```python
from build123d import *

# Parameters (mm, degrees)
SKETCH1_R               = 40
SKETCH1_R_2             = 14
BOSS_EXTRUDE1_DEPTH     = 10
SKETCH2_W               = 16
SKETCH2_H               = 60.808164115
BOSS_EXTRUDE2_DEPTH     = 10
FILLET1_R               = 4
SKETCH3_W               = 14.5
SKETCH3_H               = 2
SKETCH4_W               = 1.3
SKETCH4_H               = 0.7
CUT_EXTRUDE1_DEPTH      = 109.166538264
CUT_EXTRUDE1_DEPTH_BACK = 109.166538264
SKETCH5_W               = 2
SKETCH5_H               = 50


with BuildPart() as part:
    # Sketch1 → Boss-Extrude1 (new, symmetric)
    with BuildSketch(Plane.XY):
        Circle(SKETCH1_R)
        Circle(SKETCH1_R_2, mode=Mode.SUBTRACT)
    extrude(amount=BOSS_EXTRUDE1_DEPTH, both=True)

    # Sketch2 → Boss-Extrude2 (add, symmetric)
    with BuildSketch(Plane.XY):
        with Locations((0, 69.595917942)):
            Rectangle(SKETCH2_W, SKETCH2_H)
    extrude(amount=BOSS_EXTRUDE2_DEPTH, both=True)

    # Fillet1
    fillet1_edges = [part.edges().sort_by_distance(p)[0] for p in [
        (-8, 39.191835885, 0),
        (8, 39.191835885, 0),
    ]]
    fillet(fillet1_edges, radius=FILLET1_R)

    # Sketch3 → Cut-Revolve1 (revolve, cut)
    with BuildSketch(Plane(origin=(0, 0, 0), x_dir=(0, 0, -1), z_dir=(1, 0, 0)), mode=Mode.PRIVATE) as cut_revolve1_sk:
        with Locations((-2.75, 15)):
            Rectangle(SKETCH3_W, SKETCH3_H)
    revolve(cut_revolve1_sk.sketch.rotate(Axis((0, 0, 0), (0, 0, -1)), 90), axis=Axis((0, 0, 0), (0, 0, -1)), mode=Mode.SUBTRACT)

    # Sketch4 → Cut-Revolve2 (revolve, cut)
    with BuildSketch(Plane(origin=(0, 0, 0), x_dir=(0, 0, -1), z_dir=(1, 0, 0)), mode=Mode.PRIVATE) as cut_revolve2_sk:
        with Locations((-5.05, 16.35)):
            Rectangle(SKETCH4_W, SKETCH4_H)
    revolve(cut_revolve2_sk.sketch.rotate(Axis((0, 0, 0), (0, 0, -1)), 90), axis=Axis((0, 0, 0), (0, 0, -1)), mode=Mode.SUBTRACT)

    # Sketch5 → Cut-Extrude1 (cut, two sides: drawn at the far end of the back side and taken through both)
    with BuildSketch(Plane(origin=(0, 0, 0), x_dir=(0, 0, -1), z_dir=(1, 0, 0)).offset(-CUT_EXTRUDE1_DEPTH_BACK)):
        with Locations((9, 75)):
            Rectangle(SKETCH5_W, SKETCH5_H)
        with Locations((-9, 75)):
            Rectangle(SKETCH5_W, SKETCH5_H)
    extrude(amount=CUT_EXTRUDE1_DEPTH + CUT_EXTRUDE1_DEPTH_BACK, mode=Mode.SUBTRACT)


solid = part.part
```
Check sheet for the modelled part. Datum: model origin and axes. Units: mm. A direction names the side the tool comes from. Round coordinates to 2 decimals unless told otherwise and drop trailing zeros. Order: outer loops, then holes, each group sorted by start corner. A loop starts at its lowest first (then second) coordinate and runs counter-clockwise, first axis right, second up. Notation, with made-up numbers: (68.5, -3) -> (83.5, -3) arc R21 cw to (83.5, 8) -> close; hole circle Ø8 at (52.25, 31.25). An arc over 180 degrees is marked (long way). One line per item, written item: value. Start each with the question number.
Q1. Set-up check for faces 1 (the face through (-8, 71, 0)), 2 (the face through (0.07, 14.15, -4.5)), 3 (the face through (8, 71, 0)): record each of +Z, -Z, +X, -X, +Y, -Y from which the full face is reachable in a straight line by a thin tool's end or side.
Q2. Cross-section at C-C (y = 0). Record the boundary of the cut face in (x, z).
Q3. Cross-section at A-A (z = 1.5). Record the boundary of the cut face in (x, y), and give its area (3 significant figures).
Q4. Cross-section at B-B (x = 0). Record the boundary of the cut face in (y, z), and give its area (3 significant figures).
Q5. Cross-section at D-D (y = 58). Record the boundary of the cut face in (x, z), and give its area (3 significant figures).
Q6. Mould release check, pull along Z, two halves, no side actions. Record for faces 4 (the face through (8, 16, 10)), 5 (the face through (0, 75, -8)), 6 (the face through (-2.17, -16.56, 5.04)), 7 (the face through (-3.47, 15.62, 7.82)): pulls with the +Z half, pulls with the -Z half, needs draft (parallel to the pull), parting line crosses it, or undercut.
Q7. Thickness scan on line 1 (X direction, y = 0, z = -8.6); line 2 (Y direction, x = 0, z = 4.9); line 3 (X direction, y = 1, z = -0.25). Record the ranges inside material, lowest first.
Q8. Gauge pin test, flat ends, axial feed: pin 1 Ø6 at (y, z) = (70.5, -5) entering from +X; pin 2 Ø1 at (x, z) = (2, 9.5) entering from +Y; pin 3 Ø2 at (x, z) = (30.5, 3) entering from +Y. Record the tip position at first contact, or that the pin passes through.
Completed:
1. face 1: +Z, -Z, -X, +Y
1. face 2: +Z
1. face 3: +Z, -Z, +X, +Y
2. outline: (-40, -10) -> (-14, -10) -> (-14, -4.5) -> (-16, -4.5) -> (-16, 4.4) -> (-16.7, 4.4) -> (-16.7, 5.7) -> (-16, 5.7) -> (-16, 10) -> (-40, 10) -> close; (14, -10) -> (40, -10) -> (40, 10) -> (16, 10) -> (16, 5.7) -> (16.7, 5.7) -> (16.7, 4.4) -> (16, 4.4) -> (16, -4.5) -> (14, -4.5) -> close
3. outline: (-10.91, 38.48) arc R40 ccw (long way) to (10.91, 38.48) arc R4 cw to (8, 42.33) -> (8, 100) -> (-8, 100) -> (-8, 42.33) arc R4 cw to start; hole circle Ø32 at (0, 0)
3. area: 5,190 mm²
4. outline: (-40, -10) -> (-14, -10) -> (-14, -4.5) -> (-16, -4.5) -> (-16, 4.4) -> (-16.7, 4.4) -> (-16.7, 5.7) -> (-16, 5.7) -> (-16, 10) -> (-40, 10) -> close; (14, -10) -> (50, -10) -> (50, -8) -> (100, -8) -> (100, 8) -> (50, 8) -> (50, 10) -> (16, 10) -> (16, 5.7) -> (16.7, 5.7) -> (16.7, 4.4) -> (16, 4.4) -> (16, -4.5) -> (14, -4.5) -> close
4. area: 1,980 mm²
5. outline: (-8, -8) -> (8, -8) -> (8, 8) -> (-8, 8) -> close
5. area: 256 mm²
6. face 4: pulls with the +Z half
6. face 5: pulls with the -Z half
6. face 6: undercut
6. face 7: needs draft
7. line 1: x = -40 to -14, 14 to 40
7. line 2: y = -40 to -16.7, 16.7 to 100
7. line 3: x = -39.99 to -15.97, 15.97 to 39.99
8. pin 1: stops at x = 8
8. pin 2: stops at y = 50
8. pin 3: stops at y = 27.01
